from build123d import *


with BuildPart() as f1:
    # F0 (on Front) → F1 (revolve)
    with BuildSketch(Plane.XZ):
        with BuildLine():
            Line((7.3025, 49.9351416626), (4.7625, 49.9351416626))
            Line((4.7625, 49.9351416626), (4.7625, 40.3847416626))
            Line((4.7625, 40.3847416626), (0, 40.3847416626))
            Line((0, 40.3847416626), (0, 6.8790409714))
            Line((0, 6.8790409714), (0, 0))
            Line((0, 0), (1.5875, 0))
            Line((1.5875, 0), (1.5875, -13.5648583374))
            add(Edge.make_bspline(
                [(1.5875, -13.5648583374), (2.197826211, -11.343300191), (3.4507124513, -6.7828543454), (9.3827411245, -1.5374513186), (20.2289245805, 1.8522698942), (26.5021930747, 2.6866479243), (29.49943192, 3.0852966105)],
                knots=[0, 0, 0, 0, 0.221273734, 0.454233837, 0.7392441363, 1, 1, 1, 1], degree=3))
            ThreePointArc((29.49943192, 3.0852966105), (31.695299556, 7.825879337), (27.6678465307, 11.1537287012))
            add(Edge.make_bspline(
                [(27.6678465307, 11.1537287012), (26.2216893508, 11.2234465231), (22.8965880234, 11.3837464036), (14.647665222, 12.1059748712), (10.4700064296, 15.3881169493), (7.8159786412, 21.4408473295), (7.9325491577, 33.2367031168), (7.91835801, 38.2405007706), (7.9121207818, 40.4397472739)],
                knots=[0, 0, 0, 0, 0.1378285483, 0.3169046183, 0.456687677, 0.6146757849, 0.8306440445, 1, 1, 1, 1], degree=3))
            Line((7.9121207818, 40.4397472739), (7.9121207818, 49.8497076333))
            Line((7.9121207818, 49.8497076333), (7.3025, 49.9351416626))
        make_face()
    revolve(axis=Axis((0, 0, 20.1923708313), (0, 0, -1)))


solid = f1.part
Build history of the part. All positions in model axes, mm. A direction names the side the tool comes from. Give positions to 0.01 mm unless a question says otherwise; leave off trailing zeros. Write each loop counter-clockwise with the first axis right and the second up, starting at its lowest first coordinate (ties: lowest second). Pieces come first, ordered by that corner, then holes. Notation, with made-up numbers: (26.25, -22) - (55.25, -22) arc R10 cw to (55.25, -8) - close; hole circle Ø6 at (67.25, 20). An arc over 180 degrees is marked (long way). Use one line per item in the form item = value. Start each with the question number.
1. Probe line 1 (Y direction, x = 0, z = 45.5); line 2 (X direction, y = 3.5, z = 46). List the from-to ranges inside material, lowest first. Write a range as [from, to].
2. 3-axis set-ups, long thin cutter, end or side, ignore diameter. For faces 1 (the face through (-0.34, 1.55, -6.88)), 2 (the face through (-3.78, 2.9, 45.09)): which of +Z, -Z, +X, -X, +Y, -Y reach the whole face in a straight line?
3. Band-saw the part on A-A on z = 10. Write the cut outline in (x, y).
4. Drop flat-ended pins along their axis: pin 1 Ø5 at (x, z) = (8, 13) entering from +Y; pin 2 Ø6 at (x, y) = (7.5, 4.5) entering from -Z; pin 3 Ø3 at (x, y) = (0, 0) entering from +Z; pin 4 Ø2.5 at (x, y) = (0.5, 0.5) entering from -Z. Give the stop position or say it passes through.
5. Two-plate mould, pull along X, no slides. Class faces 3 (the face through (-7.904, -0.348, 45.211)), 4 (the face through (0, 0, 0)), 5 (the face through (5, 0, 49.935)): released by +X, released by -X, zero draft, split by the parting line, or undercut.
Conclusion:
q1.line_1 = [-7.91, -4.76], [4.76, 7.91]
q1.line_2 = [-7.1, -3.23], [3.23, 7.1]
q2.face_1 = -Z
q2.face_2 = +Z
q3.outline = circle Ø60.9 at (0, 0)
q4.pin_1 = 28.76
q4.pin_2 = -5.01
q4.pin_3 = 40.38
q4.pin_4 = -13.56
q5.face_3 = split by the parting line
q5.face_4 = undercut
q5.face_5 = zero draft
